from build123d import *

# Parameters (mm, degrees)
F1_DEPTH = 10
F2_W     = 20
F2_H     = 20
F3_DEPTH = 40
F4_R     = 1.5
F5_DEPTH = 20
F6_W     = 20
F6_H     = 20
F7_DEPTH = 10


with BuildPart() as f1:
    # F0 (on Top) → F1 (new body)
    with BuildSketch(Plane.XY):
        Polygon((-100, -10), (-100, -30), (100, -30), (100, -10), (20, -10), (20, 10), (100, 10), (100, 30), (-100, 30), (-100, 10), (-20, 10), (-20, -10), align=None)
    extrude(amount=F1_DEPTH)

    # F2 (on face) → F3 (join)
    with BuildSketch(Plane.XY.offset(10)):
        Rectangle(F2_W, F2_H)
    extrude(amount=F3_DEPTH)

    # F4 (on face) → F5 (cut)
    with BuildSketch(Plane.XZ.offset(10)):
        with Locations((0, 30)):
            Circle(F4_R)
    extrude(amount=-F5_DEPTH, mode=Mode.SUBTRACT)

    # F6 (on face) → F7 (join)
    with BuildSketch(Plane.XY.offset(50)):
        Polygon((-20, 10), (-20, -10), (-100, -10), (-100, -30), (100, -30), (100, -10), (20, -10), (20, 10), (100, 10), (100, 30), (-100, 30), (-100, 10), align=None)
        Rectangle(F6_W, F6_H, mode=Mode.SUBTRACT)
        Rectangle(F6_W, F6_H)
    extrude(amount=F7_DEPTH)


solid = f1.part
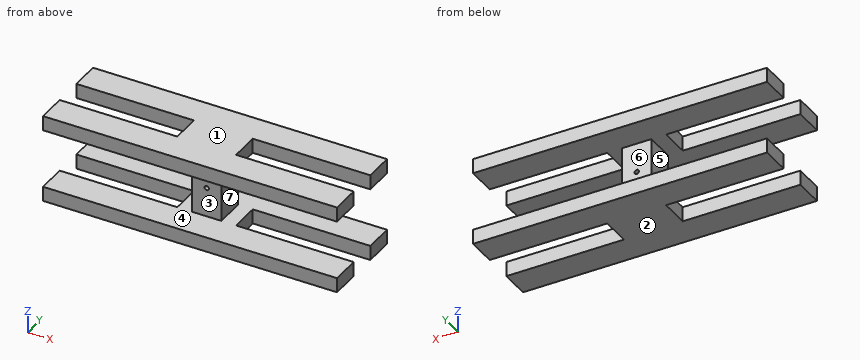
Design review of the part built by this model. Coordinates are the model's own, in mm. Face numbers are marked on the shaded views. A direction names the side the tool comes from. Give positions to 0.01 mm unless a question says otherwise; leave off trailing zeros. Loops run counter-clockwise (first coordinate to the right, second up) from the corner with the lowest first, then second, coordinate; pieces in that order, holes last. Notation, with made-up numbers: M 52.25,-8.5 L 97.25,-8.5 A16 ccw 97.25,0.5 Z; hole C -29,59 d10. An arc over 180 degrees is marked long. Write item = value, one per line.
Q1. To check wall thickness, follow line 1 (Z direction, x = -92, y = -23); line 2 (Y direction, x = -52.5, z = 9.5); line 3 (Z direction, x = 0, y = 3). State the ranges of each line that lie inside material, in increasing order. Write a range as [from, to].
Output values:
line_1 = [0, 10], [50, 60]
line_2 = [-30, -10], [10, 30]
line_3 = [0, 28.5], [31.5, 60]
Q2. Insertion check: pin 1 (16 mm diameter, centred on x = 3.5, z = 20, fed in from +Y); pin 2 (22 mm diameter, centred on y = 4.5, z = 25.5, fed in from +X); pin 3 (4 mm diameter, centred on x = 0, z = 30, fed in from -Y). Each pin has a flat end and moves straight along its axis. Give the tip position at first contact, or say it passes through.
Output values:
pin_1 = 10
pin_2 = 10
pin_3 = -10
Q3. We need section B-B (x = 3.5). Give the boundary of the cut face in (y, z), plus the area to 3 significant figures.
Output values:
outline = M -30,0 L 30,0 L 30,10 L 10,10 L 10,50 L 30,50 L 30,60 L -30,60 L -30,50 L -10,50 L -10,10 L -30,10 Z
area = 2,000 mm^2
Q4. We need section A-A (y = 3.5). Give the boundary of the cut face in (x, z).
Output values:
outline = M -20,0 L 20,0 L 20,10 L 10,10 L 10,50 L 20,50 L 20,60 L -20,60 L -20,50 L -10,50 L -10,10 L -20,10 Z; hole C 0,30 d3
Q5. We need section D-D (x = 75). Give the boundary of the cut face in (y, z), plus the area to 3 significant figures.
Output values:
outline = M -30,0 L -10,0 L -10,10 L -30,10 Z; M -30,50 L -10,50 L -10,60 L -30,60 Z; M 10,0 L 30,0 L 30,10 L 10,10 Z; M 10,50 L 30,50 L 30,60 L 10,60 Z
area = 800 mm^2
Q6. Draft analysis for pull direction Z (two halves, no side actions). For the marked faces 1, 2, 3 and 4, state which applies: +Z half, -Z half, draft (parallel to the pull), parting line (faces both ways), or undercut.
Output values:
face_1 = +Z half
face_2 = -Z half
face_3 = undercut
face_4 = undercut
Q7. For the marked faces 5, 6 and 7, list the 3-axis set-ups (+Z, -Z, +X, -X, +Y, -Y) from which the entire face can be reached by the end or side of a thin tool; tool diameter is ignored.
Output values:
face_5 = -X, +Y, -Y
face_6 = +X, -X, +Y
face_7 = +X, +Y, -Y
Q8. We need section C-C (y = 16.5). Give the boundary of the cut face in (x, z).
Output values:
outline = M -100,0 L 100,0 L 100,10 L -100,10 Z; M -100,50 L 100,50 L 100,60 L -100,60 Z
